```python
from build123d import *

# Parameters (mm, degrees)
CROQUIS1_R              = 2.38125
CROQUIS1_R_2            = 4.7625
SALIENTE_EXTRUIR1_DEPTH = 6.35


with BuildPart() as part:
    # Croquis1 → Saliente-Extruir1 (new body)
    with BuildSketch(Plane(origin=(0, 0, 0), x_dir=(1, 0, 0), z_dir=(0, 1, 0))):
        with BuildLine():
            Line((103.955940895, 6.200359073), (33.182720339, -4.250520887))
            ThreePointArc((33.182720339, -4.250520887), (31.696731466, -4.587290217), (30.279155254, -5.145908331))
            Line((30.279155254, -5.145908331), (-13.707132326, -26.482618703))
            ThreePointArc((-13.707132326, -26.482618703), (-26.984336102, -24.417368961), (-32.012638404, -11.956808276))
            ThreePointArc((-32.012638404, -11.956808276), (-30.297252372, -7.553267867), (-26.751302562, -4.429174828))
            Line((-26.751302562, -4.429174828), (8.61159414, 14.14717195))
            ThreePointArc((8.61159414, 14.14717195), (10.234533943, 14.825001148), (11.951126741, 15.208009235))
            Line((11.951126741, 15.208009235), (98.089879586, 26.598503543))
            ThreePointArc((98.089879586, 26.598503543), (103.154358957, 25.953614792), (107.240482188, 22.892825721))
            ThreePointArc((107.240482188, 22.892825721), (109.446452134, 13.78938225), (103.955940895, 6.200359073))
        make_face()
        with Locations(Location((102.277188424, 16.565289857, 0), (0, 0, 270))):
            Circle(CROQUIS1_R, mode=Mode.SUBTRACT)
        with Locations(Location((23.306287218, 3.774794841, 0), (0, 0, 270))):
            Circle(CROQUIS1_R_2, mode=Mode.SUBTRACT)
        with Locations(Location((-21.693712782, -16.225205159, 0), (0, 0, 270))):
            Circle(CROQUIS1_R, mode=Mode.SUBTRACT)
    extrude(amount=SALIENTE_EXTRUIR1_DEPTH)


solid = part.part
```
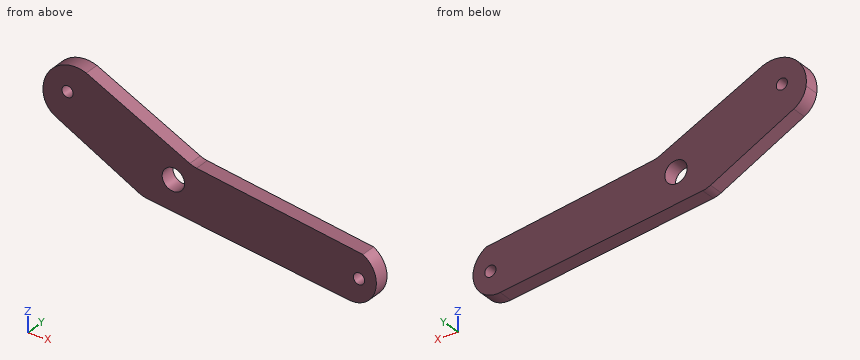
Geometry: final body of the model. Coordinates: model frame, mm. Round coordinates to 2 decimals unless told otherwise and drop trailing zeros. Loops run counter-clockwise (first coordinate to the right, second up) from the corner with the lowest first, then second, coordinate; pieces in that order, holes last. Notation, with made-up numbers: (59.5, -24.75) -> (80.5, -24.75) arc R11 ccw to (80.5, -20.75) -> close; hole circle Ø9 at (-24, 80). An arc over 180 degrees is marked (long way). Use one line per item in the form item = value. Start each with the question number.
1) Line query: L1, parallel to Z at x = 23.5, y = 2; L2, parallel to X at y = 1, z = 15.5; L3, parallel to Z at x = 103.5, y = 2. Output: solid intervals per line, ascending.
2) Section A-A on y = 1. Output: boundary loops of the cut face in (x, z) (1 decimal).
3) First-contact query: P1, Ø3, axis at x = -14, y = 1.5, coming from the -Z side; P2, Ø1, axis at y = 1, z = 12, coming from the +X side. Flat tips, straight axial feed; report the tip coordinate or a pass-through.
4) Section B-B on x = 71.5. Output: boundary loops of the cut face in (y, z).
5) Section C-C on z = 7. Output: boundary loops of the cut face in (x, y), then the cut area to 3 significant figures.
Response:
q1.L1 = -16.74 to -8.53, 0.98 to 8.43
q1.L2 = -32.02 to -23.96, -19.43 to 8.93
q1.L3 = -25.81 to -18.61, -14.52 to -6.13
q2.outline = (-32, 12) arc R10 ccw to (-26.8, 4.4) -> (8.6, -14.1) arc R10 ccw to (12, -15.2) -> (98.1, -26.6) arc R10 ccw to (107.2, -22.9) arc R11.2 ccw to (104, -6.2) -> (33.2, 4.3) arc R10 cw to (30.3, 5.1) -> (-13.7, 26.5) arc R13.6 ccw to start; hole circle Ø4.8 at (-21.7, 16.2); hole circle Ø9.5 at (23.3, -3.8); hole circle Ø4.8 at (102.3, -16.6)
q3.P1 = -3.06
q3.P2 = 17.18
q4.outline = (0, -23.08) -> (6.35, -23.08) -> (6.35, -1.41) -> (0, -1.41) -> close
q5.outline = (-29.88, 0) -> (26.46, 0) -> (26.46, 6.35) -> (-29.88, 6.35) -> close
q5.area = 358 mm^2
